Source: CAD feature listing. Evaluate the final solid. Frame: model axes, mm. Face numbers are marked on the shaded views. A direction names the side the tool comes from. Round coordinates to 2 decimals unless told otherwise and drop trailing zeros. Order: outer loops, then holes, each group sorted by start corner. A loop starts at its lowest first (then second) coordinate and runs counter-clockwise, first axis right, second up. Notation, with made-up numbers: (30.25, 18) -> (45.25, 18) arc R35 ccw to (45.25, 57) -> close; hole circle Ø2 at (54.25, 54). An arc over 180 degrees is marked (long way). Use a Markdown table: item, result. Add a question column.
Autodesk Inventor part; units mm, degrees
ref_plane "HoleTangent" through (75, 0, 0) normal (1, 0, 0) x (0, 1, 0)
ref_plane "XZ Plane" through (0, 0, 0) normal (0, 1, 0) x (-1, 0, 0)
ref_plane "XY Plane" through (0, 0, 0) normal (0, 0, 1) x (1, 0, 0)
sketch "Sketch1" plane through (0, 0, 0) normal (0, 0, 1) x (1, 0, 0)
  circle A0 centre (0, 0) radius 75
  dimension "d114" = 150
extrude "Extrusion1" add sketch "Sketch1" along normal blind 25
ref_plane "HoleTangent" through (75, 0, 0) normal (1, 0, 0) x (0, 1, 0)
sketch "Sketch3" plane through (0, 0, 25) normal (0, 0, 1) x (1, 0, 0)
  point P0 (0, 0)
  point P1 (0, 0)
hole "Hole1" at (0, 0, 25) direction (0, 0, -1) diameter 12.7 end through all
sketch "Sketch6" plane through (0, 0, 25) normal (0, 0, 1) x (1, 0, 0)
  circle A0 centre (0, 0) radius 6.35
  circle A1 centre (0, 0) radius 19.05
  dimension "d46" = 38.1
extrude "Extrusion4" cut sketch "Sketch6" against normal blind 12.5
sketch "Sketch7" plane through (0, 0, 0) normal (0, 0, -1) x (-1, 0, 0)
  circle A0 centre (0, 0) radius 6.35
  circle A1 centre (0, 0) radius 12.7 construction
  line L0 (0, 0) -> (8.9803, 8.9803) construction
  line L1 (0, 0) -> (11.1003, 0) construction
  dimension "d49" = 25.4
  dimension "d50" = 45
hole "Hole3" at (-8.9803, 8.9803, 0) direction (0, 0, 1) diameter 5.08 end through all
pattern_circular "Circular Pattern3" count 4 over 360 about axis through (0, 0, -188.6001) along (0, 0, 1) of "Hole3"
sketch "Sketch5" plane through (75, 12.7, 25.4) normal (1, 0, 0) x (0, 0, -1)
  line L0 (30.48, -12.7) -> (-5.08, -12.7)
  point P0 (12.9, -12.7)
  point P1 (25.4, -12.7)
  dimension "d116" = 12.5
hole "Hole2" at (75, 0, 12.5) direction (-1, 0, 0) diameter 12.7 depth 55.5625 counterbore diameter 15.875 counterbore depth 34.925
sketch "Sketch4" plane through (0, 0, 25) normal (0, 0, 1) x (1, 0, 0)
  line L0 (41, 18.5) -> (41, -18.5)
  line L1 (28, -18.5) -> (28, 18.5)
  arc A0 (41, 18.5) -> (28, 18.5) centre (34.5, 18.5) ccw
  arc A1 (28, -18.5) -> (41, -18.5) centre (34.5, -18.5) ccw
  circle A2 centre (0, 0) radius 19.05
  point P0 (28, 0)
  dimension "d22" = 50
  dimension "d24" = 6.5
  dimension "d62" = 34.5
extrude "Extrusion3" cut sketch "Sketch4" against normal through all contours L0 A1 L1 A0
pattern_circular "Circular Pattern2" count 3 over 360 about axis through (0, 0, -188.6001) along (0, 0, 1) of "Hole2", "Extrusion3"
sketch "Sketch8" plane through (0, 0, 25) normal (0, 0, 1) x (1, 0, 0)
  line L0 (-10.3502, -47.1424) -> (10.8733, -47.1424) construction
  line L1 (10.8733, -47.1424) -> (10.8733, -60.9041) construction
  line L2 (10.8733, -60.9041) -> (-10.3502, -60.9041) construction
  line L3 (-10.3502, -60.9041) -> (-10.3502, -47.1424) construction
  point P0 (0, 0)
hole "Hole4" at (75, 0, 12.5) direction (-1, 0, 0) diameter 22.5 depth 2
equation "\"d115\" = 0.5 * d114"
properties part number "PWTR-0032" material "Aluminum-6061"
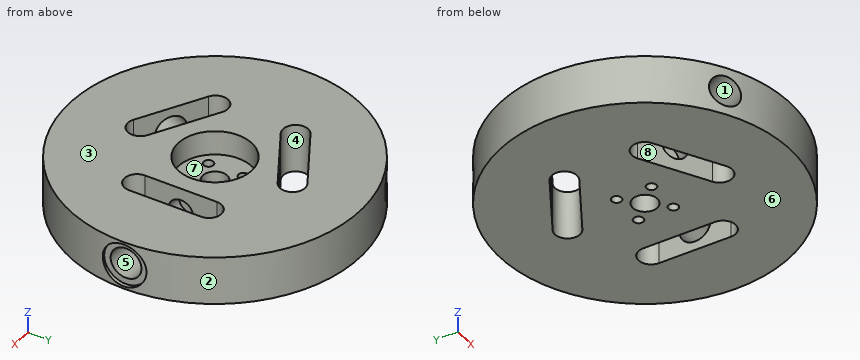
1) Draft query along X for the marked faces 1, 2, 3 and 4. Return one class per face: pulls with the +X half, pulls with the -X half, needs draft (parallel to the pull), parting line crosses it, or undercut.
2) Reachability of the marked faces 5, 6, 7 and 8 from +Z, -Z, +X, -X, +Y, -Y: full face, straight path, thin tool, end or side. Return the list, or none.
3) Section B-B on y = 29.5. Output: boundary loops of the cut face in (x, z).
4) Section D-D on z = 10.75. Count the separate pieces of the cut face and the enclosed holes in it, then the cut area to 3 significant figures.
5) Section C-C on x = 0. Output: boundary loops of the cut face in (y, z).
6) Section A-A on x = 34.5. Output: boundary loops of the cut face in (y, z), then the cut area to 3 significant figures.
7) Line query: probe 1 along Y at (x, z) = (-29, 21.25); probe 2 along Y at (x, z) = (-3, 22.25); probe 3 along Y at (x, z) = (-16, 15.75). Output: solid intervals per line, ascending. Write a range as from..to.
8) First-contact query: pin 1 Ø5 at (x, z) = (57.5, 16) entering from -Y; pin 2 Ø14.5 at (y, z) = (0, 12.5) entering from +X; pin 3 Ø4 at (y, z) = (2, 15) entering from +X. Flat tips, straight axial feed; report the tip coordinate or a pass-through.
Conclusion:
| question | item | result |
|---|---|---|
| 1 | face 1 | undercut |
| 1 | face 2 | parting line crosses it |
| 1 | face 3 | needs draft |
| 1 | face 4 | undercut |
| 2 | face 5 | +X |
| 2 | face 6 | -Z, +X, -X, +Y, -Y |
| 2 | face 7 | +Z |
| 2 | face 8 | +Z, -Z |
| 3 | outline | (-68.95, 0) -> (-30.9, 0) -> (-30.9, 25) -> (-68.95, 25) -> close; (-4.9, 0) -> (68.95, 0) -> (68.95, 25) -> (-4.9, 25) -> close |
| 4 | separate pieces | 1 |
| 4 | enclosed holes | 5 |
| 4 | area | 13,700 mm^2 |
| 5 | outline | (-75, 0) -> (-45.51, 0) -> (-45.51, 25) -> (-75, 25) -> close; (-32.33, 0) -> (-6.35, 0) -> (-6.35, 12.5) -> (-19.05, 12.5) -> (-19.05, 25) -> (-32.33, 25) -> close; (6.35, 0) -> (32.33, 0) -> (32.33, 25) -> (19.05, 25) -> (19.05, 12.5) -> (6.35, 12.5) -> close; (45.51, 0) -> (75, 0) -> (75, 25) -> (45.51, 25) -> close |
| 6 | outline | (-66.59, 0) -> (-25, 0) -> (-25, 25) -> (-66.59, 25) -> close; (25, 0) -> (66.59, 0) -> (66.59, 25) -> (25, 25) -> close |
| 6 | area | 2,080 mm^2 |
| 7 | probe 1 | y = -69.17..-30.6, -15.59..15.59, 30.6..69.17 |
| 7 | probe 2 | y = -74.94..-45.38, -30.6..-18.81, 18.81..30.6, 45.38..74.94 |
| 7 | probe 3 | y = -73.27..-42.2, -16.8..-10.34, 10.34..16.8, 42.2..73.27 |
| 8 | pin 1 | stops at y = -50.99 |
| 8 | pin 2 | stops at x = 28 |
| 8 | pin 3 | stops at x = 19.44 |
